Autodesk Inventor part; units mm, degrees
ref_plane "YZ Plane" through (0, 0, 0) normal (1, 0, 0) x (0, 1, 0)
ref_plane "XZ Plane" through (0, 0, 0) normal (0, 1, 0) x (-1, 0, 0)
ref_plane "XY Plane" through (0, 0, 0) normal (0, 0, 1) x (1, 0, 0)
sketch "Sketch2" plane through (0, 0, 0) normal (0, 1, 0) x (-1, 0, 0)
  line L0 (0, 0) -> (-59, 0)
  line L1 (-59, 0) -> (-59, 78)
  line L2 (-59, 78) -> (0, 78)
  line L3 (0, 78) -> (0, 0)
  dimension "d0" = 59
  dimension "d1" = 78
extrude "Extrusion1" add sketch "Sketch2" along normal blind 45
shell "Shell1" thickness 3 removed faces 1 at (39.3333, 45, 52)
sketch "Sketch4" plane through (59, 0, 0) normal (0, 0, -1) x (-1, 0, 0)
  point P0 (59, 0)
sketch "Sketch5" plane through (3, 3, 3) normal (0, 0, 1) x (1, 0, 0)
  line L0 (0, 0) -> (0, 42)
  line L1 (0, 42) -> (53, 42)
  line L2 (0, 0) -> (53, 0)
  line L3 (53, 0) -> (53, 42)
  line L4 (53, 42) -> (0, 42)
  line L5 (0, 42) -> (0, 0)
  point P0 (-3, -3)
extrude "Extrusion3" cut sketch "Sketch5" against normal blind 10
sketch "Sketch6" plane through (0, 0, 0) normal (-1, 0, 0) x (0, 0, 1)
  line L0 (4.5, 37.5) -> (30.5, 37.5)
  line L1 (30.5, 37.5) -> (30.5, 33.5)
  line L2 (30.5, 33.5) -> (4.5, 33.5)
  line L3 (4.5, 33.5) -> (4.5, 37.5)
  line L4 (0, 0) -> (0, 45)
  line L5 (0, 0) -> (78, 0)
  dimension "d19" = 26
  dimension "d20" = 4
  dimension "d21" = 4.5
  dimension "d22" = 33.5
sketch "Sketch7" plane through (59, 0, 78) normal (1, 0, 0) x (0, 0, -1)
  line L0 (0, 0) -> (78, 0)
  line L1 (0, 45) -> (78, 45)
  line L2 (78, 45) -> (78, 0)
  line L3 (78, 0) -> (0, 0)
  line L4 (0, 0) -> (0, 45)
extrude "Extrusion5" add sketch "Sketch7" along normal blind 3
extrude "Extrusion6" cut sketch "Sketch6" against normal through all
sketch "Sketch8" plane through (0, 0, 0) normal (-1, 0, 0) x (0, 0, 1)
  circle A0 centre (50, 35.5) radius 2.5
  point P0 (0, 0)
  dimension "d29" = 5
extrude "Extrusion7" cut sketch "Sketch8" against normal through all
properties part number "arduino with shield box v05"
Build history of the part. All positions in model axes, mm. A direction names the side the tool comes from. Round coordinates to 2 decimals unless told otherwise and drop trailing zeros. Write each loop counter-clockwise with the first axis right and the second up, starting at its lowest first coordinate (ties: lowest second). Pieces come first, ordered by that corner, then holes. Notation, with made-up numbers: (-2.5, -37.75) -> (46.5, -37.75) arc R30 cw to (46.5, -7.75) -> close; hole circle Ø4 at (30, 43). An arc over 180 degrees is marked (long way). Use one line per item in the form item = value.
Q1. Band-saw the part on B-B, the plane y = 35.5. Write the cut outline in (x, z).
Conclusion:
outline = (0, 0) -> (3, 0) -> (3, 4.5) -> (0, 4.5) -> close; (0, 30.5) -> (3, 30.5) -> (3, 47.5) -> (0, 47.5) -> close; (0, 52.5) -> (3, 52.5) -> (3, 75) -> (56, 75) -> (56, 52.5) -> (62, 52.5) -> (62, 78) -> (0, 78) -> close; (56, 0) -> (62, 0) -> (62, 4.5) -> (56, 4.5) -> close; (56, 30.5) -> (62, 30.5) -> (62, 47.5) -> (56, 47.5) -> close
Q2. Band-saw the part on D-D, the plane z = 65. Write the cut outline in (x, y).
Conclusion:
outline = (0, 0) -> (62, 0) -> (62, 45) -> (56, 45) -> (56, 3) -> (3, 3) -> (3, 45) -> (0, 45) -> close
Q3. Band-saw the part on C-C, the plane x = 46. Write the cut outline in (y, z), then the cut area to 3 significant figures.
Conclusion:
outline = (0, 0) -> (3, 0) -> (3, 75) -> (45, 75) -> (45, 78) -> (0, 78) -> close
area = 360 mm²
Q4. Two-plate mould, pull along X, no slides. Class faces 4 (the flat face through (59, 33.5, 18)), 5 (the flat face through (29, 3, 38)), 6 (the flat face through (0, 22, 40)): released by +X, released by -X, zero draft, split by the parting line, or undercut.
Conclusion:
face_4 = zero draft
face_5 = undercut
face_6 = released by -X
Q5. Band-saw the part on A-A, the plane z = 50. Write the cut outline in (x, y).
Conclusion:
outline = (0, 0) -> (62, 0) -> (62, 33) -> (56, 33) -> (56, 3) -> (3, 3) -> (3, 33) -> (0, 33) -> close; (0, 38) -> (3, 38) -> (3, 45) -> (0, 45) -> close; (56, 38) -> (62, 38) -> (62, 45) -> (56, 45) -> close
Q6. Drill centre lines: L1, parallel to Y at x = 59, z = 50; L2, parallel to X at y = 27.5, z = 39; L3, parallel to Y at x = 59, z = 28. Where is each one in solid material? Low to high.
Conclusion:
L1 = 0 to 33, 38 to 45
L2 = 0 to 3, 56 to 62
L3 = 0 to 33.5, 37.5 to 45
Q7. Drop flat-ended pins along their axis: P1, Ø2, axis at x = 15.5, z = 67, coming from the +Y side; P2, Ø21, axis at x = 32, y = 23, coming from the -Z side. Give the stop position or say it passes through.
Conclusion:
P1 = 3
P2 = 75
Q8. Tool access for faces 1 (the flat face through (1, 33.5, 18)), 2 (the flat face through (30, 24, 75)), 3 (the flat face through (31, 0, 40)): list every direction of +Z, -Z, +X, -X, +Y, -Y with a clear straight run to the whole face (end or side of a thin tool).
Conclusion:
face_1 = +X, -X
face_2 = -Z, +Y
face_3 = +Z, -Z, +X, -X, -Y
